Verification items for the finished model (mm, model axes). A direction names the side the tool comes from. Coordinates: 2 decimals unless noted, no trailing zeros. Order: outer loops, then holes, each group sorted by start corner. A loop starts at its lowest first (then second) coordinate and runs counter-clockwise, first axis right, second up. Notation, with made-up numbers: M 28,-9 L 52,-9 A13 ccw 52,12 Z; hole C -3.75,31 d6. An arc over 180 degrees is marked long. Write item = value, one per line.
```python
from build123d import *

# Parameters (mm, degrees)
SKETCH1_R           = 12.5
BOSS_EXTRUDE1_DEPTH = 25
SKETCH2_R           = 11.5
CUT_EXTRUDE1_DEPTH  = 24
CUT_EXTRUDE2_REACH  = 32.619
SKETCH3_R           = 1
CHAMFER1_SIZE       = 1


with BuildPart() as part:
    # Sketch1 → Boss-Extrude1 (new body)
    with BuildSketch(Plane(origin=(0, 0, 0), x_dir=(1, 0, 0), z_dir=(0, 1, 0))):
        with Locations(Location((0, 0, 0), (0, 0, 270))):
            Circle(SKETCH1_R)
    extrude(amount=BOSS_EXTRUDE1_DEPTH)

    # Sketch2 → Cut-Extrude1 (cut)
    with BuildSketch(Plane(origin=(0, 25, 0), x_dir=(1, 0, 0), z_dir=(0, 1, 0))):
        with Locations(Location((0, 0, 0), (0, 0, 270))):
            Circle(SKETCH2_R)
    extrude(amount=-CUT_EXTRUDE1_DEPTH, mode=Mode.SUBTRACT)

    # Sketch3 → Cut-Extrude2 (cut, up to next)
    with BuildSketch(Plane.XZ, mode=Mode.PRIVATE) as cut_extrude2_sk1:
        with Locations(Location((0, 0, 0), (0, 0, 270))):
            Circle(SKETCH3_R)
    cut_extrude2_tool1 = extrude(cut_extrude2_sk1.sketch, amount=-CUT_EXTRUDE2_REACH, mode=Mode.PRIVATE) & part.part
    # Sketch3 → Cut-Extrude2 (cut, up to next)
    with BuildSketch(Plane.XZ, mode=Mode.PRIVATE) as cut_extrude2_sk2:
        with Locations(Location((-2.828427125, 2.828427125, 0), (0, 0, 270))):
            Circle(SKETCH3_R)
    cut_extrude2_tool2 = extrude(cut_extrude2_sk2.sketch, amount=-CUT_EXTRUDE2_REACH, mode=Mode.PRIVATE) & part.part
    # Sketch3 → Cut-Extrude2 (cut, up to next)
    with BuildSketch(Plane.XZ, mode=Mode.PRIVATE) as cut_extrude2_sk3:
        with Locations(Location((-5.656854249, 5.656854249, 0), (0, 0, 270))):
            Circle(SKETCH3_R)
    cut_extrude2_tool3 = extrude(cut_extrude2_sk3.sketch, amount=-CUT_EXTRUDE2_REACH, mode=Mode.PRIVATE) & part.part
    # Sketch3 → Cut-Extrude2 (cut, up to next)
    with BuildSketch(Plane.XZ, mode=Mode.PRIVATE) as cut_extrude2_sk4:
        with Locations(Location((0, 8, 0), (0, 0, 270))):
            Circle(SKETCH3_R)
    cut_extrude2_tool4 = extrude(cut_extrude2_sk4.sketch, amount=-CUT_EXTRUDE2_REACH, mode=Mode.PRIVATE) & part.part
    # Sketch3 → Cut-Extrude2 (cut, up to next)
    with BuildSketch(Plane.XZ, mode=Mode.PRIVATE) as cut_extrude2_sk5:
        with Locations(Location((0, 4, 0), (0, 0, 270))):
            Circle(SKETCH3_R)
    cut_extrude2_tool5 = extrude(cut_extrude2_sk5.sketch, amount=-CUT_EXTRUDE2_REACH, mode=Mode.PRIVATE) & part.part
    # Sketch3 → Cut-Extrude2 (cut, up to next)
    with BuildSketch(Plane.XZ, mode=Mode.PRIVATE) as cut_extrude2_sk6:
        with Locations(Location((2.828427125, 2.828427125, 0), (0, 0, 270))):
            Circle(SKETCH3_R)
    cut_extrude2_tool6 = extrude(cut_extrude2_sk6.sketch, amount=-CUT_EXTRUDE2_REACH, mode=Mode.PRIVATE) & part.part
    # Sketch3 → Cut-Extrude2 (cut, up to next)
    with BuildSketch(Plane.XZ, mode=Mode.PRIVATE) as cut_extrude2_sk7:
        with Locations(Location((5.656854249, 5.656854249, 0), (0, 0, 270))):
            Circle(SKETCH3_R)
    cut_extrude2_tool7 = extrude(cut_extrude2_sk7.sketch, amount=-CUT_EXTRUDE2_REACH, mode=Mode.PRIVATE) & part.part
    # Sketch3 → Cut-Extrude2 (cut, up to next)
    with BuildSketch(Plane.XZ, mode=Mode.PRIVATE) as cut_extrude2_sk8:
        with Locations(Location((8, 0, 0), (0, 0, 270))):
            Circle(SKETCH3_R)
    cut_extrude2_tool8 = extrude(cut_extrude2_sk8.sketch, amount=-CUT_EXTRUDE2_REACH, mode=Mode.PRIVATE) & part.part
    # Sketch3 → Cut-Extrude2 (cut, up to next)
    with BuildSketch(Plane.XZ, mode=Mode.PRIVATE) as cut_extrude2_sk9:
        with Locations(Location((4, 0, 0), (0, 0, 270))):
            Circle(SKETCH3_R)
    cut_extrude2_tool9 = extrude(cut_extrude2_sk9.sketch, amount=-CUT_EXTRUDE2_REACH, mode=Mode.PRIVATE) & part.part
    # Sketch3 → Cut-Extrude2 (cut, up to next)
    with BuildSketch(Plane.XZ, mode=Mode.PRIVATE) as cut_extrude2_sk10:
        with Locations(Location((2.828427125, -2.828427125, 0), (0, 0, 270))):
            Circle(SKETCH3_R)
    cut_extrude2_tool10 = extrude(cut_extrude2_sk10.sketch, amount=-CUT_EXTRUDE2_REACH, mode=Mode.PRIVATE) & part.part
    # Sketch3 → Cut-Extrude2 (cut, up to next)
    with BuildSketch(Plane.XZ, mode=Mode.PRIVATE) as cut_extrude2_sk11:
        with Locations(Location((5.656854249, -5.656854249, 0), (0, 0, 270))):
            Circle(SKETCH3_R)
    cut_extrude2_tool11 = extrude(cut_extrude2_sk11.sketch, amount=-CUT_EXTRUDE2_REACH, mode=Mode.PRIVATE) & part.part
    # Sketch3 → Cut-Extrude2 (cut, up to next)
    with BuildSketch(Plane.XZ, mode=Mode.PRIVATE) as cut_extrude2_sk12:
        with Locations(Location((0, -4, 0), (0, 0, 270))):
            Circle(SKETCH3_R)
    cut_extrude2_tool12 = extrude(cut_extrude2_sk12.sketch, amount=-CUT_EXTRUDE2_REACH, mode=Mode.PRIVATE) & part.part
    # Sketch3 → Cut-Extrude2 (cut, up to next)
    with BuildSketch(Plane.XZ, mode=Mode.PRIVATE) as cut_extrude2_sk13:
        with Locations(Location((-2.828427125, -2.828427125, 0), (0, 0, 270))):
            Circle(SKETCH3_R)
    cut_extrude2_tool13 = extrude(cut_extrude2_sk13.sketch, amount=-CUT_EXTRUDE2_REACH, mode=Mode.PRIVATE) & part.part
    # Sketch3 → Cut-Extrude2 (cut, up to next)
    with BuildSketch(Plane.XZ, mode=Mode.PRIVATE) as cut_extrude2_sk14:
        with Locations(Location((-4, 0, 0), (0, 0, 270))):
            Circle(SKETCH3_R)
    cut_extrude2_tool14 = extrude(cut_extrude2_sk14.sketch, amount=-CUT_EXTRUDE2_REACH, mode=Mode.PRIVATE) & part.part
    # Sketch3 → Cut-Extrude2 (cut, up to next)
    with BuildSketch(Plane.XZ, mode=Mode.PRIVATE) as cut_extrude2_sk15:
        with Locations(Location((-8, 0, 0), (0, 0, 270))):
            Circle(SKETCH3_R)
    cut_extrude2_tool15 = extrude(cut_extrude2_sk15.sketch, amount=-CUT_EXTRUDE2_REACH, mode=Mode.PRIVATE) & part.part
    # Sketch3 → Cut-Extrude2 (cut, up to next)
    with BuildSketch(Plane.XZ, mode=Mode.PRIVATE) as cut_extrude2_sk16:
        with Locations(Location((-5.656854249, -5.656854249, 0), (0, 0, 270))):
            Circle(SKETCH3_R)
    cut_extrude2_tool16 = extrude(cut_extrude2_sk16.sketch, amount=-CUT_EXTRUDE2_REACH, mode=Mode.PRIVATE) & part.part
    # Sketch3 → Cut-Extrude2 (cut, up to next)
    with BuildSketch(Plane.XZ, mode=Mode.PRIVATE) as cut_extrude2_sk17:
        with Locations(Location((0, -8, 0), (0, 0, 270))):
            Circle(SKETCH3_R)
    cut_extrude2_tool17 = extrude(cut_extrude2_sk17.sketch, amount=-CUT_EXTRUDE2_REACH, mode=Mode.PRIVATE) & part.part
    add(cut_extrude2_tool1.solids().sort_by_distance((0, 0, 0))[0], mode=Mode.SUBTRACT)
    add(cut_extrude2_tool2.solids().sort_by_distance((-2.828427, 0, 2.828427))[0], mode=Mode.SUBTRACT)
    add(cut_extrude2_tool3.solids().sort_by_distance((-5.656854, 0, 5.656854))[0], mode=Mode.SUBTRACT)
    add(cut_extrude2_tool4.solids().sort_by_distance((0, 0, 8))[0], mode=Mode.SUBTRACT)
    add(cut_extrude2_tool5.solids().sort_by_distance((0, 0, 4))[0], mode=Mode.SUBTRACT)
    add(cut_extrude2_tool6.solids().sort_by_distance((2.828427, 0, 2.828427))[0], mode=Mode.SUBTRACT)
    add(cut_extrude2_tool7.solids().sort_by_distance((5.656854, 0, 5.656854))[0], mode=Mode.SUBTRACT)
    add(cut_extrude2_tool8.solids().sort_by_distance((8, 0, 0))[0], mode=Mode.SUBTRACT)
    add(cut_extrude2_tool9.solids().sort_by_distance((4, 0, 0))[0], mode=Mode.SUBTRACT)
    add(cut_extrude2_tool10.solids().sort_by_distance((2.828427, 0, -2.828427))[0], mode=Mode.SUBTRACT)
    add(cut_extrude2_tool11.solids().sort_by_distance((5.656854, 0, -5.656854))[0], mode=Mode.SUBTRACT)
    add(cut_extrude2_tool12.solids().sort_by_distance((0, 0, -4))[0], mode=Mode.SUBTRACT)
    add(cut_extrude2_tool13.solids().sort_by_distance((-2.828427, 0, -2.828427))[0], mode=Mode.SUBTRACT)
    add(cut_extrude2_tool14.solids().sort_by_distance((-4, 0, 0))[0], mode=Mode.SUBTRACT)
    add(cut_extrude2_tool15.solids().sort_by_distance((-8, 0, 0))[0], mode=Mode.SUBTRACT)
    add(cut_extrude2_tool16.solids().sort_by_distance((-5.656854, 0, -5.656854))[0], mode=Mode.SUBTRACT)
    add(cut_extrude2_tool17.solids().sort_by_distance((0, 0, -8))[0], mode=Mode.SUBTRACT)

    # Chamfer1
    chamfer1_edges = [part.edges().sort_by_distance(p)[0] for p in [
        (0, 0, -12.5),
        (0, 1, -11.5),
    ]]
    chamfer(chamfer1_edges, length=CHAMFER1_SIZE)


solid = part.part
```
Item 1: Sectioned sample at A-A, the plane y = 21.75. Enter the section's corners in (x, z).
Report:
outline = C 0,0 d25; hole C 0,0 d23
Item 2: Sectioned sample at B-B, the plane x = 2.25. Give the number of separate pieces and of enclosed holes in the cut face, then the cut area to 3 significant figures.
Report:
separate_pieces = 3
enclosed_holes = 0
area = 70.2 mm^2
Item 3: Tool access check on faces 1 (the cylindrical face through (5.05, 0.49, 6.45)), 2 (the cylindrical face through (9.7, 13.66, 6.18)). Record the directions out of +Z, -Z, +X, -X, +Y, -Y that give a thin tool (end or side, any length) a straight path to the whole face; none if there is none.
Report:
face_1 = +Y, -Y
face_2 = +Y
Item 4: Release check for a two-part mould opening along Z. For faces 3 (the cylindrical face through (3.755, 12.832, 11.923)), 4 (the flat face through (0, 0, 2)), 5 (the cylindrical face through (-7.01, 0.49, 0.13)) record: pulls with the +Z half, pulls with the -Z half, needs draft (parallel to the pull), parting line crosses it, or undercut.
Report:
face_3 = parting line crosses it
face_4 = needs draft
face_5 = undercut
Item 5: Scan lines: L1, parallel to Y at x = -1, z = -9; L2, parallel to Z at x = 4, y = 5.75; L3, parallel to X at y = 20.25, z = -8. Record each from-to range of solid material in increasing order. Write a range as from..to.
Report:
L1 = 0..1
L2 = -11.84..-10.78, 10.78..11.84
L3 = -9.6..-8.26, 8.26..9.6
Item 6: Gauge pin test, flat ends, axial feed: pin 1 (1.6 mm diameter, centred on x = 0, z = 4, fed in from +Y); pin 2 (2.5 mm diameter, centred on x = 0, z = -4, fed in from +Y); pin 3 (1.5 mm diameter, centred on y = 7.5, z = 1.5, fed in from -X); pin 4 (8 mm diameter, centred on y = 3, z = -7, fed in from +X). Record the tip position at first contact, or that the pin passes through.
Report:
pin_1 = through
pin_2 = 1
pin_3 = -12.48
pin_4 = 12.13
